CAD build for the part. Positions are in the model's coordinates, mm. A direction names the side the tool comes from. Round coordinates to 2 decimals unless told otherwise and drop trailing zeros. Order: outer loops, then holes, each group sorted by start corner. A loop starts at its lowest first (then second) coordinate and runs counter-clockwise, first axis right, second up. Notation, with made-up numbers: M -27.5,-34 L 1.5,-34 A15 ccw 1.5,-23 Z; hole C 3,57.25 d2. An arc over 180 degrees is marked long. Answer as a JSON object with one key per item and string values. Group by question number.
```python
from build123d import *

# Parameters (mm, degrees)
F0_R     = 2
F1_DEPTH = 15
F2_DEPTH = 3
F3_R     = 5
F4_R     = 5
F5_R     = 1.2


with BuildPart() as f1:
    # F0 (on Top) → F1 (new body)
    with BuildSketch(Plane.XY):
        with BuildLine():
            Line((9.5707826587, -1.8608114628), (7.3763099499, 0))
            ThreePointArc((7.3763099499, 0), (5.2158387857, -5.2158387857), (0, -7.3763099499))
            Line((0, -7.3763099499), (2.2002961183, -9.4984839312))
            ThreePointArc((2.2002961183, -9.4984839312), (7.0159164816, -6.770481218), (9.5707826587, -1.8608114628))
        make_face()
        with BuildLine():
            ThreePointArc((0, -7.3763099499), (5.2158387857, -5.2158387857), (7.3763099499, 0))
            ThreePointArc((7.3763099499, 0), (5.2158387857, 5.2158387857), (0, 7.3763099499))
            ThreePointArc((0, 7.3763099499), (-5.2158387857, 5.2158387857), (-7.3763099499, 0))
            ThreePointArc((-7.3763099499, 0), (-5.2158387857, -5.2158387857), (0, -7.3763099499))
        make_face()
        Circle(F0_R, mode=Mode.SUBTRACT)
        with BuildLine():
            ThreePointArc((9.5742217065, 1.8430351908), (7.7357792995, 5.9346624697), (4.2599529151, 8.7701368952))
            Line((4.2599529151, 8.7701368952), (1.7095643673, 9.02517575))
            Line((1.7095643673, 9.02517575), (0, 7.3763099499))
            ThreePointArc((0, 7.3763099499), (5.2158387857, 5.2158387857), (7.3763099499, 0))
            Line((7.3763099499, 0), (9.5742217065, 1.8430351908))
        make_face()
        with BuildLine():
            Line((1.7095643673, 9.02517575), (4.2599529151, 8.7701368952))
            ThreePointArc((4.2599529151, 8.7701368952), (3.2505886766, 9.1921800056), (2.2002961183, 9.4984839312))
            Line((2.2002961183, 9.4984839312), (1.7095643673, 9.02517575))
        make_face()
        with BuildLine():
            Line((-1.7095643673, 9.02517575), (-4.2599529151, 8.7701368952))
            ThreePointArc((-4.2599529151, 8.7701368952), (-7.7357792995, 5.9346624697), (-9.5742217065, 1.8430351908))
            Line((-9.5742217065, 1.8430351908), (-7.3763099499, 0))
            ThreePointArc((-7.3763099499, 0), (-5.2158387857, 5.2158387857), (0, 7.3763099499))
            Line((0, 7.3763099499), (-1.7095643673, 9.02517575))
        make_face()
        with BuildLine():
            ThreePointArc((-2.2002961183, 9.4984839312), (-3.2505886766, 9.1921800056), (-4.2599529151, 8.7701368952))
            Line((-4.2599529151, 8.7701368952), (-1.7095643673, 9.02517575))
            Line((-1.7095643673, 9.02517575), (-2.2002961183, 9.4984839312))
        make_face()
        with BuildLine():
            Line((-7.3763099499, 0), (-9.5707826587, -1.8608114628))
            ThreePointArc((-9.5707826587, -1.8608114628), (-7.0159164816, -6.770481218), (-2.2002961183, -9.4984839312))
            Line((-2.2002961183, -9.4984839312), (0, -7.3763099499))
            ThreePointArc((0, -7.3763099499), (-5.2158387857, -5.2158387857), (-7.3763099499, 0))
        make_face()
    extrude(amount=F1_DEPTH)

    # F0 (on Top) → F2 (join)
    with BuildSketch(Plane.XY):
        with BuildLine():
            Line((4.2599529151, 8.7701368952), (10.7868960269, 8.1174425841))
            ThreePointArc((10.7868960269, 8.1174425841), (0, 13.5), (-10.7868960269, 8.1174425841))
            Line((-10.7868960269, 8.1174425841), (-4.2599529151, 8.7701368952))
            ThreePointArc((-4.2599529151, 8.7701368952), (-3.2505886766, 9.1921800056), (-2.2002961183, 9.4984839312))
            ThreePointArc((-2.2002961183, 9.4984839312), (0, 9.75), (2.2002961183, 9.4984839312))
            ThreePointArc((2.2002961183, 9.4984839312), (3.2505886766, 9.1921800056), (4.2599529151, 8.7701368952))
        make_face()
        Polygon((0, 7.3763099499), (1.7095643673, 9.02517575), (0, 9.1961321867), (-1.7095643673, 9.02517575), align=None)
        with BuildLine():
            Line((1.7095643673, 9.02517575), (2.2002961183, 9.4984839312))
            ThreePointArc((2.2002961183, 9.4984839312), (0, 9.75), (-2.2002961183, 9.4984839312))
            Line((-2.2002961183, 9.4984839312), (-1.7095643673, 9.02517575))
            Line((-1.7095643673, 9.02517575), (0, 9.1961321867))
            Line((0, 9.1961321867), (1.7095643673, 9.02517575))
        make_face()
        with BuildLine():
            ThreePointArc((8.2654431298, -10.6739144585), (12.1209216286, -5.9441785701), (13.5, 0))
            ThreePointArc((13.5, 0), (12.8037708579, 4.2794219024), (10.7868960269, 8.1174425841))
            Line((10.7868960269, 8.1174425841), (4.2599529151, 8.7701368952))
            ThreePointArc((4.2599529151, 8.7701368952), (7.7357792995, 5.9346624697), (9.5742217065, 1.8430351908))
            ThreePointArc((9.5742217065, 1.8430351908), (9.7059559457, 0.9256992928), (9.75, 0))
            ThreePointArc((9.75, 0), (9.7050922438, -0.9347109387), (9.5707826587, -1.8608114628))
            ThreePointArc((9.5707826587, -1.8608114628), (7.0159164816, -6.770481218), (2.2002961183, -9.4984839312))
            ThreePointArc((2.2002961183, -9.4984839312), (0, -9.75), (-2.2002961183, -9.4984839312))
            ThreePointArc((-2.2002961183, -9.4984839312), (-7.0159164816, -6.770481218), (-9.5707826587, -1.8608114628))
            ThreePointArc((-9.5707826587, -1.8608114628), (-9.7499957971, -0.0090529401), (-9.5742217065, 1.8430351908))
            ThreePointArc((-9.5742217065, 1.8430351908), (-7.7357792995, 5.9346624697), (-4.2599529151, 8.7701368952))
            Line((-4.2599529151, 8.7701368952), (-10.7868960269, 8.1174425841))
            ThreePointArc((-10.7868960269, 8.1174425841), (-13.3800852655, -1.7953602115), (-8.2654431298, -10.6739144585))
            Line((-8.2654431298, -10.6739144585), (0, -9.8038678133))
            Line((0, -9.8038678133), (8.2654431298, -10.6739144585))
        make_face()
        with BuildLine():
            ThreePointArc((-8.2654431298, -10.6739144585), (-13.3800852655, -1.7953602115), (-10.7868960269, 8.1174425841))
            Line((-10.7868960269, 8.1174425841), (-20, 7.1961321867))
            ThreePointArc((-20, 7.1961321867), (-17.9538534771, -2.2224916805), (-19, -11.8038678133))
            Line((-19, -11.8038678133), (-8.2654431298, -10.6739144585))
        make_face()
        with BuildLine():
            ThreePointArc((-6.5512368792, -11.8038678133), (-7.4298519681, -11.2715260605), (-8.2654431298, -10.6739144585))
            Line((-8.2654431298, -10.6739144585), (-19, -11.8038678133))
            Line((-19, -11.8038678133), (-6.5512368792, -11.8038678133))
        make_face()
        with BuildLine():
            Line((19, -11.8038678133), (8.2654431298, -10.6739144585))
            ThreePointArc((8.2654431298, -10.6739144585), (7.4298519681, -11.2715260605), (6.5512368792, -11.8038678133))
            Line((6.5512368792, -11.8038678133), (19, -11.8038678133))
        make_face()
        with BuildLine():
            ThreePointArc((6.5512368792, -11.8038678133), (7.4298519681, -11.2715260605), (8.2654431298, -10.6739144585))
            Line((8.2654431298, -10.6739144585), (0, -9.8038678133))
            Line((0, -9.8038678133), (-8.2654431298, -10.6739144585))
            ThreePointArc((-8.2654431298, -10.6739144585), (-7.4298519681, -11.2715260605), (-6.5512368792, -11.8038678133))
            Line((-6.5512368792, -11.8038678133), (6.5512368792, -11.8038678133))
        make_face()
        with BuildLine():
            ThreePointArc((10.7868960269, 8.1174425841), (12.8037708579, 4.2794219024), (13.5, 0))
            ThreePointArc((13.5, 0), (12.1209216286, -5.9441785701), (8.2654431298, -10.6739144585))
            Line((8.2654431298, -10.6739144585), (19, -11.8038678133))
            ThreePointArc((19, -11.8038678133), (17.9538534771, -2.2224916805), (20, 7.1961321867))
            Line((20, 7.1961321867), (10.7868960269, 8.1174425841))
        make_face()
        with BuildLine():
            ThreePointArc((9.75, 0), (9.7059559457, 0.9256992928), (9.5742217065, 1.8430351908))
            Line((9.5742217065, 1.8430351908), (7.3763099499, 0))
            Line((7.3763099499, 0), (9.5707826587, -1.8608114628))
            ThreePointArc((9.5707826587, -1.8608114628), (9.7050922438, -0.9347109387), (9.75, 0))
        make_face()
        with BuildLine():
            Line((-7.3763099499, 0), (-9.5742217065, 1.8430351908))
            ThreePointArc((-9.5742217065, 1.8430351908), (-9.7499957971, -0.0090529401), (-9.5707826587, -1.8608114628))
            Line((-9.5707826587, -1.8608114628), (-7.3763099499, 0))
        make_face()
        with BuildLine():
            Line((2.2002961183, -9.4984839312), (0, -7.3763099499))
            Line((0, -7.3763099499), (-2.2002961183, -9.4984839312))
            ThreePointArc((-2.2002961183, -9.4984839312), (0, -9.75), (2.2002961183, -9.4984839312))
        make_face()
    extrude(amount=F2_DEPTH)

    # F3
    f3_edges = [f1.edges().sort_by_distance(p)[0] for p in [
        (19, -11.803868, 1.5),
    ]]
    fillet(f3_edges, radius=F3_R)

    # F4
    f4_edges = [f1.edges().sort_by_distance(p)[0] for p in [
        (-19, -11.803868, 1.5),
        (20, 7.196132, 1.5),
        (-20, 7.196132, 1.5),
    ]]
    fillet(f4_edges, radius=F4_R)

    # F5
    f5_edges = [f1.edges().sort_by_distance(p)[0] for p in [
        (0, -11.803868, 3),
        (0, 13.5, 3),
        (0, -11.803868, 0),
        (0, 13.5, 0),
    ]]
    fillet(f5_edges, radius=F5_R)


solid = f1.part
```
Item 1: 3-axis set-ups, long thin cutter, end or side, ignore diameter. For faces 1 (the face through (-8.46, -0.92, 8.92)), 2 (the face through (8.489, -0.943, 8.916)), 3 (the face through (0, -9, 3)), 4 (the face through (6.96, -6.83, 8.92)), 5 (the face through (-7.07, -6.714, 8.916)): which of +Z, -Z, +X, -X, +Y, -Y reach the whole face in a straight line?
Item 2: Two-plate mould, pull along X, no slides. Class faces 6 (the face through (-16.686, -10.227, 1.504)), 7 (the face through (0, -2, 7)), 8 (the face through (16.8, -10.1, 1.5)): +X half, -X half, draft (parallel to the pull), parting line (faces both ways), or undercut.
Item 3: Flat gauge pins, fed straight in: pin 1 Ø6 at (x, y) = (-14.5, -7) entering from +Z; pin 2 Ø5 at (x, z) = (-5, 12.5) entering from +Y; pin 3 Ø1 at (x, z) = (-4, 12) entering from -Y. Where does each tip first touch, or does it go through?
Item 4: Cut at A-A, the plane z = 5.5. Give the cut face in (x, y), and give its area (3 significant figures).
Item 5: Drill centre lines: line 1 (X direction, y = 8.75, z = 3.5); line 2 (Z direction, x = -1, y = -10.25); line 3 (X direction, y = -8.5, z = 12.25). Where is each one in solid material? Low to high. Write a range as [from, to].
Response values:
{
 "1": {"face 1": "+Z, -X", "face 2": "+Z, +X", "face 3": "+Z", "face 4": "+Z, +X, -Y", "face 5": "+Z, -X, -Y"},
 "2": {"face 6": "-X half", "face 7": "undercut", "face 8": "+X half"},
 "3": {"pin 1": "z = 3", "pin 2": "y = 9.42", "pin 3": "y = -9.1"},
 "4": {"outline": "M -9.57,-1.86 A9.75 ccw -2.2,-9.5 L 0,-7.38 L 2.2,-9.5 A9.75 ccw 9.57,-1.86 L 7.38,0 L 9.57,1.84 A9.75 ccw 2.2,9.5 L 0,7.38 L -2.2,9.5 A9.75 ccw -9.57,1.84 L -7.38,0 Z; hole C 0,0 d4", "area": "266 mm^2"},
 "5": {"line 1": "[-4.3, -1.42], [1.42, 4.3]", "line 2": "[0, 3]", "line 3": "[-4.78, -1.17], [1.17, 4.78]"}
}
